CAD build for the part. Positions are in the model's coordinates, mm. A direction names the side the tool comes from. Give positions to 0.01 mm unless a question says otherwise; leave off trailing zeros. Loops run counter-clockwise (first coordinate to the right, second up) from the corner with the lowest first, then second, coordinate; pieces in that order, holes last.
Autodesk Inventor part; units mm, degrees
ref_plane "YZ Plane" through (0, 0, 0) normal (1, 0, 0) x (0, 1, 0)
ref_plane "XZ Plane" through (0, 0, 0) normal (0, 1, 0) x (-1, 0, 0)
ref_plane "XY Plane" through (0, 0, 0) normal (0, 0, 1) x (1, 0, 0)
sketch "Sketch1" plane through (0, 0, 0) normal (0, 1, 0) x (-1, 0, 0)
  line L0 (0, 0) -> (145, 0)
  line L1 (145, 0) -> (145, -30)
  line L2 (145, -30) -> (0, -30)
  line L3 (0, -30) -> (0, 0)
  line L4 (145, 0) -> (115, 0)
  line L5 (115, 0) -> (115, -70)
  line L6 (115, -70) -> (145, -70)
  line L7 (145, -70) -> (145, 0)
  point P0 (115, -30)
  dimension "d0" = 145
  dimension "d1" = 30
  dimension "d2" = 30
  dimension "d3" = 70
extrude "Extrusion1" add sketch "Sketch1" along normal blind 30
sketch "Sketch2" plane through (0, 0, -30) normal (0, 0, -1) x (-1, 0, 0)
  line L0 (0, 20) -> (135, 20)
  line L1 (135, 20) -> (135, 10)
  line L2 (135, 10) -> (0, 10)
  line L3 (0, 10) -> (0, 20)
  dimension "d32" = 135
  dimension "d33" = 10
extrude "Extrusion2" cut sketch "Sketch2" along normal blind 50 and the other way blind 20
sketch "Sketch4" plane through (0, 30, 0) normal (0, 1, 0) x (1, 0, 0)
  line L0 (0, 0) -> (-145, 0)
  line L1 (-145, 0) -> (-145, 10)
  line L2 (-145, 10) -> (0, 10)
  line L3 (0, 10) -> (0, 0)
  line L4 (-115, 70) -> (-145, 70)
  line L5 (-145, 70) -> (-135, 70)
  line L6 (-135, 70) -> (-135, 10)
  line L7 (-135, 10) -> (-145, 10)
  line L8 (-145, 10) -> (-145, 70)
  line L9 (-115, 30) -> (-115, 70)
  line L10 (-115, 70) -> (-125, 70)
  line L11 (-125, 70) -> (-125, 30)
  line L12 (-125, 30) -> (-115, 30)
  line L13 (-115, 30) -> (-115, 70)
  line L14 (0, 30) -> (-125, 30)
  line L15 (-125, 30) -> (-125, 20)
  line L16 (-125, 20) -> (0, 20)
  line L17 (0, 20) -> (0, 30)
  dimension "d22" = 145
  dimension "d23" = 10
  dimension "d24" = 10
  dimension "d25" = 60
  dimension "d26" = 10
  dimension "d27" = 40
  dimension "d28" = 125
  dimension "d29" = 10
extrude "Extrusion4" add sketch "Sketch4" along normal blind 20
properties part number "TSU_Corner1_Clamp"
1. Tool access for faces 1 (the face through (-67, 15, -10)), 2 (the face through (-68, 40, -10)), 3 (the face through (-135, 40, -40)), 4 (the face through (-94, 50, -9)), 5 (the face through (-58, 5, -30)): list every direction of +Z, -Z, +X, -X, +Y, -Y with a clear straight run to the whole face (end or side of a thin tool).
Responses:
face 1: -Z, +X
face 2: +X, +Y
face 3: -Z, +Y
face 4: +Z, -Z, +X, -X, +Y
face 5: -Z, +X, +Y, -Y
2. Saw through at C-C, the plane z = -12. List the corners of the cut face in (x, y), and give its area (3 significant figures).
Responses:
outline: (-145, 0) - (0, 0) - (0, 10) - (-135, 10) - (-135, 20) - (0, 20) - (0, 30) - (-135, 30) - (-135, 50) - (-145, 50) - close
area: 3,200 mm2
3. Saw through at A-A, the plane x = -122.5. List the corners of the cut face in (y, z).
Responses:
outline: (0, -70) - (10, -70) - (10, -10) - (20, -10) - (20, -70) - (50, -70) - (50, -20) - (30, -20) - (30, -10) - (50, -10) - (50, 0) - (0, 0) - close
4. Pull direction Z, two halves, no side cores. Call faces 6 (the face through (-63, 40, -20)), 7 (the face through (-130, 25, -70)), 8 (the face through (-125, 40, -45)): released by +Z, released by -Z, zero draft, split by the parting line, or undercut.
Responses:
face 6: undercut
face 7: released by -Z
face 8: zero draft
5. Probe line 1 along Y through (x, z) = (-117.5, -32); line 2 along Y through (x, z) = (-17.5, -12); line 3 along X through (y, z) = (42, -64). List the from-to ranges inside material, lowest first.
Responses:
line 1: y = 0 to 10, 20 to 50
line 2: y = 0 to 10, 20 to 30
line 3: x = -145 to -135, -125 to -115
6. Saw through at D-D, the plane z = -33. List the corners of the cut face in (x, y).
Responses:
outline: (-145, 0) - (-115, 0) - (-115, 10) - (-135, 10) - (-135, 20) - (-115, 20) - (-115, 50) - (-125, 50) - (-125, 30) - (-135, 30) - (-135, 50) - (-145, 50) - close
7. Drop flat-ended pins along their axis: pin 1 (4 mm diameter, centred on x = -81, z = -16.5, fed in from -Y); pin 2 (24 mm diameter, centred on x = -37.5, y = 41.5, fed in from -Z); pin 3 (2 mm diameter, centred on x = -85.5, z = -18, fed in from +Y); pin 4 (8 mm diameter, centred on y = 3, z = -46.5, fed in from +X). Give the stop position or say it passes through.
Responses:
pin 1: stops at y = 0
pin 2: stops at z = -30
pin 3: stops at y = 30
pin 4: stops at x = -115
8. Saw through at B-B, the plane y = 26. List the corners of the cut face in (x, z).
Responses:
outline: (-145, -70) - (-115, -70) - (-115, -30) - (0, -30) - (0, 0) - (-145, 0) - close
